The model under review builds one solid part; all positions refer to its coordinate system, in mm. Face numbers are marked on the shaded views. A direction names the side the tool comes from. Give positions to 0.01 mm unless a question says otherwise; leave off trailing zeros. Order: outer loops, then holes, each group sorted by start corner. A loop starts at its lowest first (then second) coordinate and runs counter-clockwise, first axis right, second up. Notation, with made-up numbers: M 47,44.5 L 102,44.5 A23 cw 102,79.5 Z; hole C -28,-38.75 d1. An arc over 180 degrees is marked long. One line per question, with ' | ' between items. Start each with the question number.
1. We need section D-D on x = 5.5. Write out the cut boundary in (y, z), then the cut area to 3 significant figures.
2. Insertion check: P1, Ø8, axis at y = 55, z = 5, coming from the +X side; P2, Ø6, axis at x = -5.5, y = 20, coming from the +Z side; P3, Ø5.5, axis at y = 107.5, z = -1.5, coming from the -X side. Each pin has a flat end and moves straight along its axis. Give the tip position at first contact, or say it passes through.
3. We need section A-A on x = 0. Write out the cut boundary in (y, z).
4. For the marked faces 1, 2 and 3, list the 3-axis set-ups (+Z, -Z, +X, -X, +Y, -Y) from which the entire face can be reached by the end or side of a thin tool; tool diameter is ignored.
5. Wall thickness on L1, parallel to Y at x = 3.5, z = 2.75; L2, parallel to X at y = 11.5, z = -3; L3, parallel to Z at x = 2.5, y = 72.5: over which ranges is each line inside the solid? List them lowest first.
6. We need section C-C on y = 27.5. Write out the cut boundary in (x, z), then the cut area to 3 significant figures.
7. We need section B-B on z = 0. Write out the cut boundary in (x, y), then the cut area to 4 significant figures.
```python
from build123d import *

# Parameters (mm, degrees)
CUT_EXTRUDE1_DEPTH = 5
CUT_EXTRUDE2_DEPTH = 99
FILLET1_R          = 1


with BuildPart() as part:
    # Sketch5 → Revolve1 (revolve)
    with BuildSketch(Plane.XY, mode=Mode.PRIVATE) as revolve1_sk:
        Polygon((0, 0), (7.25, 0), (7.25, 5), (5, 5), (5, 104), (4.5, 109), (0, 109), align=None)
    revolve(revolve1_sk.sketch.rotate(Axis((0, 109, 0), (0, -1, 0)), 180), axis=Axis((0, 109, 0), (0, -1, 0)))

    # Sketch6 → Cut-Extrude1 (cut)
    with BuildSketch(Plane(origin=(0, 109, 0), x_dir=(1, 0, 0), z_dir=(0, 1, 0))):
        with BuildLine():
            Line((3, 4), (3, -4))
            ThreePointArc((3, -4), (5, 0), (3, 4))
        make_face()
        with BuildLine():
            Line((-3, 4), (-3, -4))
            ThreePointArc((-3, -4), (-5, 0), (-3, 4))
        make_face()
    extrude(amount=-CUT_EXTRUDE1_DEPTH, mode=Mode.SUBTRACT)

    # Sketch7 → Cut-Extrude2 (cut)
    with BuildSketch(Plane(origin=(0, 104, 0), x_dir=(1, 0, 0), z_dir=(0, 1, 0))):
        with BuildLine():
            Line((3, -4), (3, 4))
            ThreePointArc((3, 4), (5, 0), (3, -4))
        make_face()
    extrude(amount=-CUT_EXTRUDE2_DEPTH, mode=Mode.SUBTRACT)

    # Fillet1
    # the kernel refuses this fillet: 1 mm, written as the material it takes off along each edge
    with BuildSketch(Plane(origin=(3, 108.493644566, 4), x_dir=(0, 0, -1), z_dir=(0, -1, 0))) as fillet1_piece_1:
        with BuildLine():
            CenterArc((0.535898385, -1), FILLET1_R, 90, 60)
            ThreePointArc((-0.330127019, -0.5), (-0.172559651, -0.245050643), (0, 0))
            Line((0, 0), (0.535898385, 0))
        make_face()
    extrude(amount=103.493644566, mode=Mode.SUBTRACT)
    with BuildSketch(Plane(origin=(3, 108.493644566, -4), x_dir=(0, 0, 1), z_dir=(0, -1, 0))) as fillet1_piece_2:
        with BuildLine():
            CenterArc((0.535898385, 1), FILLET1_R, 210, 60)
            ThreePointArc((-0.330127019, 0.5), (-0.172559651, 0.245050643), (0, 0))
            Line((0, 0), (0.535898385, 0))
        make_face()
    extrude(amount=103.493644566, mode=Mode.SUBTRACT)


solid = part.part
```
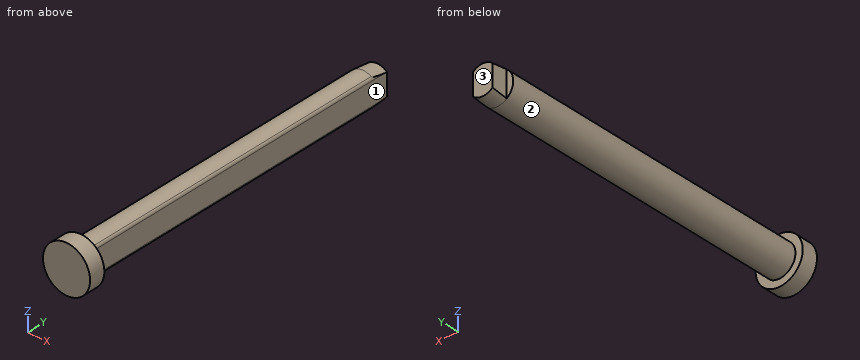
Entries:
1) outline: M 0,-4.72 L 5,-4.72 L 5,4.72 L 0,4.72 Z | area: 47.2 mm^2
2) P1: stops at x = 3 | P2: stops at z = 4.33 | P3: stops at x = -3
3) outline: M 0,-7.25 L 5,-7.25 L 5,-5 L 104,-5 L 109,-4.5 L 109,4.5 L 104,5 L 5,5 L 5,7.25 L 0,7.25 Z
4) face 1: +Z, -Z, +X, +Y | face 2: +Y | face 3: +Z, -Z, +X, -X, +Y
5) L1: y = 0 to 5 | L2: x = -4 to 3 | L3: z = -4.33 to 4.33
6) outline: M 2.5,-4.33 A1 ccw 3,-3.46 L 3,3.46 A1 ccw 2.5,4.33 A5 ccw long Z | area: 67.3 mm^2
7) outline: M -7.25,0 L 7.25,0 L 7.25,5 L 3,5 L 3,109 L -3,109 L -3,104 L -5,104 L -5,5 L -7.25,5 Z | area: 894.5 mm^2
